```python
from build123d import *

# Parameters (mm, degrees)
SKETCH1_W                    = 76.2
SKETCH1_H                    = 127
BOSS_EXTRUDE1_DEPTH          = 24.13
SKETCH2_R                    = 7.9375
F_1_2_13_THREADED_HOLE_DEPTH = 78.885280381
SKETCH3_R                    = 5.0419
F_3_8_THROUGH_HOLES_DEPTH    = 78.885280381


with BuildPart() as part:
    # Sketch1 → Boss-Extrude1 (new body)
    with BuildSketch(Plane(origin=(0, 0, 0), x_dir=(1, 0, 0), z_dir=(0, 1, 0))):
        Rectangle(SKETCH1_W, SKETCH1_H)
    extrude(amount=BOSS_EXTRUDE1_DEPTH)

    # Sketch2 → 1/2"-13 Threaded Hole (cut, through all)
    with BuildSketch(Plane(origin=(0, 24.13, 0), x_dir=(1, 0, 0), z_dir=(0, 1, 0))):
        with Locations(Location((0, 0, 0), (0, 0, 270))):
            Circle(SKETCH2_R)
    extrude(amount=-F_1_2_13_THREADED_HOLE_DEPTH, mode=Mode.SUBTRACT)

    # Sketch3 → 3/8" Through Holes (cut, through all)
    with BuildSketch(Plane(origin=(0, 24.13, 0), x_dir=(1, 0, 0), z_dir=(0, 1, 0))):
        with Locations(Location((-19.05, 44.45, 0), (0, 0, 270))):
            Circle(SKETCH3_R)
        with Locations(Location((19.05, 44.45, 0), (0, 0, 270))):
            Circle(SKETCH3_R)
        with Locations(Location((19.05, -44.45, 0), (0, 0, 270))):
            Circle(SKETCH3_R)
        with Locations(Location((-19.05, -44.45, 0), (0, 0, 270))):
            Circle(SKETCH3_R)
    extrude(amount=-F_3_8_THROUGH_HOLES_DEPTH, mode=Mode.SUBTRACT)


solid = part.part
```
Check sheet for the modelled part. Datum: model origin and axes. Units: mm. Round coordinates to 2 decimals unless told otherwise and drop trailing zeros. Loops run counter-clockwise (first coordinate to the right, second up) from the corner with the lowest first, then second, coordinate; pieces in that order, holes last. Notation, with made-up numbers: (74, 44.25) - (82, 44.25) arc R20 ccw to (82, 52.25) - close; hole circle Ø11 at (-3, 58). An arc over 180 degrees is marked (long way). Write item = value, one per line. Start each with the question number.
Q1. Thickness scan on L1, parallel to X at y = 15, z = -44.45; L2, parallel to Z at x = -19.5, y = 7.5; L3, parallel to Z at x = -15.5, y = 19.5. Record the ranges inside material, lowest first.
Q2. Section check C-C (y = 5.75). Count the separate pieces of the cut face and the enclosed holes in it, plus the area to 3 significant figures.
Q3. Release check for a two-part mould opening along Z. For faces 1 (the face through (-18.828, 12.234, 39.413)), 2 (the face through (-1, 12, -63.5)), 3 (the face through (-9, 24.13, -1)) record: pulls with the +Z half, pulls with the -Z half, needs draft (parallel to the pull), parting line crosses it, or undercut.
Q4. Section check B-B (z = 44.45). Record the boundary of the cut face in (x, y), plus the area to 3 significant figures.
Q5. Section check D-D (x = 19.05). Record the boundary of the cut face in (y, z), plus the area to 3 significant figures.
Q6. Section check A-A (x = 0). Record the boundary of the cut face in (y, z), plus the area to 3 significant figures.
Q7. Depth check by flat-ended pin: P1, Ø12.5, axis at x = 0, z = 0, coming from the -Y side (1 decimal). Enter the tip coordinate at first touch or a pass-through.
Derived:
q1.L1 = -38.1 to -24.09, -14.01 to 14.01, 24.09 to 38.1
q1.L2 = -63.5 to -49.47, -39.43 to 39.43, 49.47 to 63.5
q1.L3 = -63.5 to -48.03, -40.87 to 40.87, 48.03 to 63.5
q2.separate_pieces = 1
q2.enclosed_holes = 5
q2.area = 9,160 mm^2
q3.face_1 = undercut
q3.face_2 = pulls with the -Z half
q3.face_3 = needs draft
q4.outline = (-38.1, 0) - (-24.09, 0) - (-24.09, 24.13) - (-38.1, 24.13) - close; (-14.01, 0) - (14.01, 0) - (14.01, 24.13) - (-14.01, 24.13) - close; (24.09, 0) - (38.1, 0) - (38.1, 24.13) - (24.09, 24.13) - close
q4.area = 1,350 mm^2
q5.outline = (0, -63.5) - (24.13, -63.5) - (24.13, -49.49) - (0, -49.49) - close; (0, -39.41) - (24.13, -39.41) - (24.13, 39.41) - (0, 39.41) - close; (0, 49.49) - (24.13, 49.49) - (24.13, 63.5) - (0, 63.5) - close
q5.area = 2,580 mm^2
q6.outline = (0, -63.5) - (24.13, -63.5) - (24.13, -7.94) - (0, -7.94) - close; (0, 7.94) - (24.13, 7.94) - (24.13, 63.5) - (0, 63.5) - close
q6.area = 2,680 mm^2
q7.P1 = through
